from build123d import *

# Parameters (mm, degrees)
ESBO_O1_R                = 11
ESBO_O1_R_2              = 1.75
ESBO_O1_R_3              = 2.75
RESSALTO_EXTRUS_O1_DEPTH = 7
CORTE_EXTRUS_O5_DEPTH    = 4
ESBO_O12_R               = 1.75
CORTE_EXTRUS_O6_DEPTH    = 3.5
PADR_OCIRCULAR1_COUNT    = 2


with BuildPart() as part:
    # Esboço1 → Ressalto-extrusão1 (new body)
    with BuildSketch(Plane.XY):
        Circle(ESBO_O1_R)
        with Locations((5.656854249, 5.656854249)):
            Circle(ESBO_O1_R_2, mode=Mode.SUBTRACT)
        with Locations((-5.656854249, -5.656854249)):
            Circle(ESBO_O1_R_2, mode=Mode.SUBTRACT)
        Circle(ESBO_O1_R_3, mode=Mode.SUBTRACT)
    extrude(amount=RESSALTO_EXTRUS_O1_DEPTH)

    # Esboço10 → Corte-extrusão5 (cut)
    with BuildSketch(Plane.XY.offset(7)):
        Polygon((-1.195433963, -4.461420287), (3.265986324, -3.265986324), (4.461420287, 1.195433963), (1.195433963, 4.461420287), (-3.265986324, 3.265986324), (-4.461420287, -1.195433963), align=None)
    extrude(amount=-CORTE_EXTRUS_O5_DEPTH, mode=Mode.SUBTRACT)

    # Esboço12 → Corte-extrusão6 (cut)
    with BuildSketch(Plane(origin=(0, 0, 0), x_dir=(-1, 0, 0), z_dir=(0, 0, -1))):
        with BuildLine():
            ThreePointArc((-7.954951288, 3.358757211), (-3.358757211, 3.358757211), (-3.358757211, 7.954951288))
            Line((-3.358757211, 7.954951288), (-5.132834935, 9.729029013))
            ThreePointArc((-5.132834935, 9.729029013), (-7.778174593, 7.778174593), (-9.729029013, 5.132834935))
            Line((-9.729029013, 5.132834935), (-7.954951288, 3.358757211))
        make_face()
        with Locations(Location((-5.656854249, 5.656854249, 0), (0, 0, 180))):
            Circle(ESBO_O12_R, mode=Mode.SUBTRACT)
    corte_extrus_o6 = extrude(amount=-CORTE_EXTRUS_O6_DEPTH, mode=Mode.SUBTRACT)

    # PadrãoCircular1: Corte-extrusão6 ×2 about axis
    padr_ocircular1_axis = Axis((0, 0, 0), (0, 0, 1))
    for i in range(1, PADR_OCIRCULAR1_COUNT):
        add(corte_extrus_o6.rotate(padr_ocircular1_axis, i * 360 / PADR_OCIRCULAR1_COUNT), mode=Mode.SUBTRACT)


solid = part.part
Read the model definition and answer for the solid it produces. Units are mm, in the model's axes. A direction names the side the tool comes from. Round coordinates to 2 decimals unless told otherwise and drop trailing zeros. Loops run counter-clockwise (first coordinate to the right, second up) from the corner with the lowest first, then second, coordinate; pieces in that order, holes last.
Q1. Section D-D on z = 5 is taken. Write down the section's boundary in (x, y).
Q2. Section B-B on x = -6.75 is taken. Write down the section's boundary in (y, z).
Q3. Which of the six approach directions +Z, -Z, +X, -X, +Y, -Y give full straight-line access (tool end or side, diameter ignored) to faces 5 (the face through (-4.233, -8.83, 1.726)), 6 (the face through (7.273, 4.987, 5.226)), 7 (the face through (2.3, -2.3, 0)), 8 (the face through (-3.855, 1.067, 5.028)), 9 (the face through (-6, -8, 3.5))?
Q4. Each of these flat-tipped pins is pushed along its axis until it touches: pin 1 (5.5 mm diameter, centred on x = -5.66, y = -5.66, fed in from +Z); pin 2 (1 mm diameter, centred on y = -8.5, z = 3.5, fed in from +X); pin 3 (2.5 mm diameter, centred on x = 2, y = 1.5, fed in from +Z); pin 4 (4 mm diameter, centred on x = 5.66, y = 5.66, fed in from -Z). Where does it stop, or does it pass through?
Q5. Determine the mould class of faces 1 (the face through (8.854, 4.258, 1.726)), 2 (the face through (-8.854, -4.258, 1.726)), 3 (the face through (4.233, 8.83, 1.726)), 4 (the face through (5.076, -9.759, 3.451)) for opening direction Y: released by +Y, released by -Y, zero draft, split by the parting line, or undercut.
Q6. Consider probe 1 along X at (y, z) = (0, 1.35); probe 2 along Z at (x, y) = (-8.5, -6.25); probe 3 along X at (y, z) = (2.5, 6.5). Determine where each line is inside the solid, lowest interval first.
Output:
1. outline: circle Ø22 at (0, 0); hole circle Ø3.5 at (-5.66, -5.66); hole (-4.46, -1.2) - (-1.2, -4.46) - (3.27, -3.27) - (4.46, 1.2) - (1.2, 4.46) - (-3.27, 3.27) - close; hole circle Ø3.5 at (5.66, 5.66)
2. outline: (-8.69, 3.5) - (-7.02, 3.5) - (-7.02, 7) - (-8.69, 7) - close; (-4.29, 3.5) - (-2.6, 3.5) - (-2.6, 0) - (8.69, 0) - (8.69, 7) - (-4.29, 7) - close
3. face 5: -Z, -X
3. face 6: +Z, -Z
3. face 7: -Z, +X, -X, +Y, -Y
3. face 8: +Z
3. face 9: -Z
4. pin 1: stops at z = 7
4. pin 2: stops at x = 7.55
4. pin 3: stops at z = 3
4. pin 4: stops at z = 3.5
5. face 1: released by +Y
5. face 2: released by -Y
5. face 3: undercut
5. face 4: split by the parting line
6. probe 1: x = -11 to -2.75, 2.75 to 11
6. probe 2: z = 3.5 to 7
6. probe 3: x = -10.71 to -3.47, 3.16 to 10.71
